Source: CAD feature listing. Evaluate the final solid. Frame: model axes, mm. Round coordinates to 2 decimals unless told otherwise and drop trailing zeros. Order: outer loops, then holes, each group sorted by start corner. A loop starts at its lowest first (then second) coordinate and runs counter-clockwise, first axis right, second up. Notation, with made-up numbers: M 16,-15 L 35,-15 A28 cw 35,12 Z; hole C -6,33 d7. An arc over 180 degrees is marked long. Answer as CSV lines item,"result". Start each with the question number.
Item 1: Section query C-C on z = 346.45. Return the cut outline in (x, y).
Item 2: First-contact query: P1, Ø2.5, axis at x = 319, z = 348.5, coming from the -Y side. Flat tip, straight axial feed; report the tip coordinate or a pass-through.
Item 3: Line query: line 1 (X direction, y = 789, z = 348.7); line 2 (Y direction, x = 208.5, z = 347.85); line 3 (Y direction, x = 283.5, z = 345.8). Output: solid intervals per line, ascending. Write a range as [from, to].
Item 4: Section query B-B on x = 214. Return the cut outline in (y, z), plus the area to 4 significant figures.
Item 5: Section query A-A on y = 745. Return the cut outline in (x, z).
from build123d import *

# Parameters (mm, degrees)
BOSS_EXTRUDE1_DEPTH = 400
SKETCH2_W           = 100
SKETCH2_H           = 121
SKETCH2_W_2         = 95.3
SKETCH2_H_2         = 9.4
CUT_EXTRUDE1_DEPTH  = 268
CUT_EXTRUDE2_DEPTH  = 574
CUT_EXTRUDE3_DEPTH  = 574


with BuildPart() as part:
    # Sketch1 → Boss-Extrude1 (new body)
    with BuildSketch(Plane(origin=(0, 0, 0), x_dir=(0, 0, -1), z_dir=(1, 0, 0))):
        with BuildLine():
            Line((0, 0), (-350, 0))
            Line((-350, 0), (-350, 860))
            ThreePointArc((-350, 860), (-338.284271247, 888.284271247), (-310, 900))
            Line((-310, 900), (-158.48888922, 900))
            Line((-158.48888922, 900), (-158.48888922, 1060.696902422))
            ThreePointArc((-158.48888922, 1060.696902422), (-46.288149621, 1012.851918963), (0, 900))
            Line((0, 900), (0, 0))
        make_face()
    extrude(amount=BOSS_EXTRUDE1_DEPTH)

    # Sketch2 → Cut-Extrude1 (cut)
    with BuildSketch(Plane.XY.offset(350)):
        with Locations((200, 789.5)):
            Rectangle(SKETCH2_W, SKETCH2_H)
        with Locations((325, 789.5)):
            Rectangle(SKETCH2_W_2, SKETCH2_H_2)
    extrude(amount=-CUT_EXTRUDE1_DEPTH, mode=Mode.SUBTRACT)

    # Sketch3 → Cut-Extrude2 (cut)
    with BuildSketch(Plane.ZY):
        Polygon((350, 860), (345, 860), (345, -140.268205657), (-654.048621222, 0), (-155.382910131, 1729.32315512), (878.315397885, 1431.24705506), align=None)
    extrude(amount=-CUT_EXTRUDE2_DEPTH, mode=Mode.SUBTRACT)

    # Sketch4 → Cut-Extrude3 (cut)
    with BuildSketch(Plane.XY.offset(350)):
        with BuildLine():
            Line((15, 917.971493868), (15, 330))
            ThreePointArc((15, 330), (35.502525317, 280.502525317), (85, 260))
            Line((85, 260), (315, 260))
            ThreePointArc((315, 260), (364.497474683, 280.502525317), (385, 330))
            Line((385, 330), (385, 917.971493868))
            Line((385, 917.971493868), (580.540592228, 679.226510724))
            Line((580.540592228, 679.226510724), (899.548672457, -163.886240254))
            Line((899.548672457, -163.886240254), (163.483674451, -163.886240254))
            Line((163.483674451, -163.886240254), (110.907603164, -163.886240254))
            Line((110.907603164, -163.886240254), (-601.64880395, 753.812426605))
            Line((-601.64880395, 753.812426605), (15, 917.971493868))
        make_face()
    extrude(amount=-CUT_EXTRUDE3_DEPTH, mode=Mode.SUBTRACT)


solid = part.part
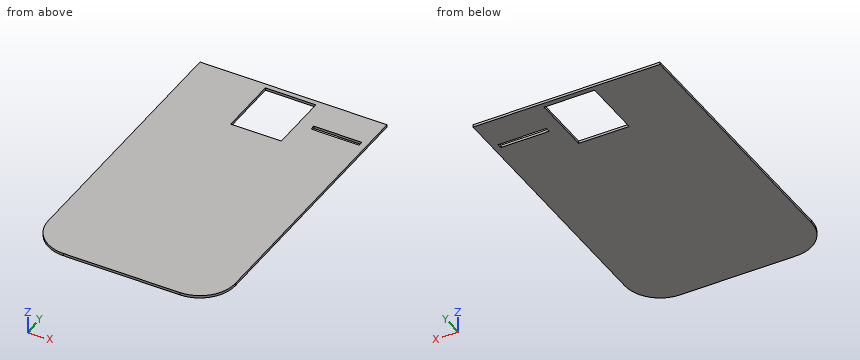
Results:
1,outline,"M 15,330 A70 ccw 85,260 L 315,260 A70 ccw 385,330 L 385,860 L 15,860 Z; hole M 150,729 L 250,729 L 250,850 L 150,850 Z; hole M 277.35,784.8 L 372.65,784.8 L 372.65,794.2 L 277.35,794.2 Z"
2,P1,"y = 260.05"
3,line 1,"[15, 150], [250, 277.35], [372.65, 385]"
3,line 2,"[260, 729], [850, 860]"
3,line 3,"[260, 784.8], [794.2, 860]"
4,outline,"M 260,345 L 729,345 L 729,350 L 260,350 Z; M 850,345 L 860,345 L 860,350 L 850,350 Z"
4,area,"2,395 mm^2"
5,outline,"M 15,345 L 150,345 L 150,350 L 15,350 Z; M 250,345 L 385,345 L 385,350 L 250,350 Z"
